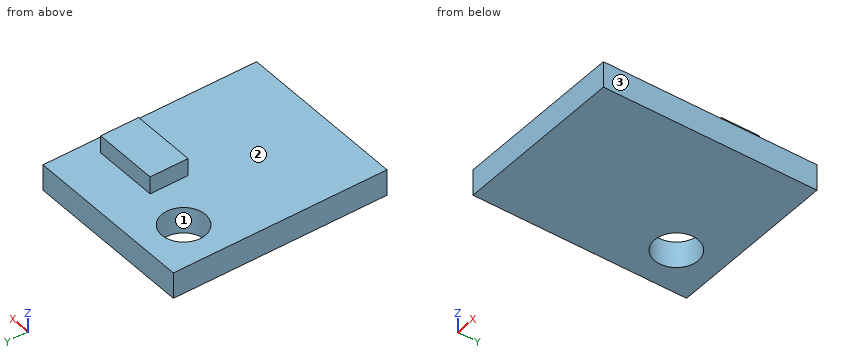
Autodesk Inventor part; units mm, degrees
ref_plane "YZ Plane" through (0, 0, 0) normal (1, 0, 0) x (0, 1, 0)
ref_plane "XZ Plane" through (0, 0, 0) normal (0, 1, 0) x (-1, 0, 0)
ref_plane "XY Plane" through (0, 0, 0) normal (0, 0, 1) x (1, 0, 0)
sketch "Sketch1" plane through (0, 0, 0) normal (0, 0, 1) x (1, 0, 0)
  line L0 (-7.75, 4.08) -> (3.05, 4.08)
  line L1 (3.05, 4.08) -> (3.05, -9.42)
  line L2 (3.05, -9.42) -> (-7.75, -9.42)
  line L3 (-7.75, -9.42) -> (-7.75, 4.08)
  circle A0 centre (-5.025, 1.355) radius 1.375
  line L4 (-2.05, 1.2) -> (2.05, 1.2)
  line L5 (2.05, 1.2) -> (2.05, -1.2)
  line L6 (2.05, -1.2) -> (-2.05, -1.2)
  line L7 (-2.05, -1.2) -> (-2.05, 1.2)
  line L8 (-2.05, 0) -> (2.05, 0)
  line L9 (0, 1.2) -> (0, 0)
  dimension "d0" = 10.8
  dimension "d1" = 13.5
  dimension "d3" = 2.725
  dimension "d4" = 2.75
  dimension "d5" = 4.1
  dimension "d6" = 2.4
  dimension "d8" = 2.88
  dimension "d13" = 1
  dimension "d14" = 2.725
extrude "Extrusion1" add sketch "Sketch1" along normal blind 1.65
extrude "Extrusion2" add sketch "Sketch1" along normal blind 2.75 contours L4 L9 L8 L7 | L4 L5 L8 L9 | L8 L5 L6 L7
properties part number "VL53LDK"
Read the model definition and answer for the solid it produces. Units are mm, in the model's axes. Face numbers are marked on the shaded views. Coordinates: 2 decimals unless noted, no trailing zeros. Loops run counter-clockwise (first coordinate to the right, second up) from the corner with the lowest first, then second, coordinate; pieces in that order, holes last. Notation, with made-up numbers: (4.25, 42.5) - (45.25, 42.5) arc R22 cw to (45.25, 69.5) - close; hole circle Ø6 at (-22.75, 71.5). An arc over 180 degrees is marked (long way). Answer in a Markdown table with one row per item.
1. Find section D-D, the plane y = -1. Write down the section's boundary in (x, z), then the cut area to 3 significant figures.
Conclusion:
| item | result |
|---|---|
| outline | (-7.75, 0) - (3.05, 0) - (3.05, 1.65) - (2.05, 1.65) - (2.05, 2.75) - (-2.05, 2.75) - (-2.05, 1.65) - (-7.75, 1.65) - close |
| area | 22.3 mm² |
2. Find section A-A, the plane x = -1.5. Write down the section's boundary in (y, z), then the cut area to 3 significant figures.
Conclusion:
| item | result |
|---|---|
| outline | (-9.42, 0) - (4.08, 0) - (4.08, 1.65) - (1.2, 1.65) - (1.2, 2.75) - (-1.2, 2.75) - (-1.2, 1.65) - (-9.42, 1.65) - close |
| area | 24.9 mm² |
3. Straight lines are drawn through the part: line 1 (Z direction, x = 0, y = -6); line 2 (Y direction, x = 1.75, z = 1.75); line 3 (X direction, y = -1, z = 2). For each, find the intervals that lie inside material, in ascending order.
Conclusion:
| item | result |
|---|---|
| line 1 | z = 0 to 1.65 |
| line 2 | y = -1.2 to 1.2 |
| line 3 | x = -2.05 to 2.05 |
4. Find section B-B, the plane y = 2. Write down the section's boundary in (x, z), then the cut area to 3 significant figures.
Conclusion:
| item | result |
|---|---|
| outline | (-7.75, 0) - (-6.24, 0) - (-6.24, 1.65) - (-7.75, 1.65) - close; (-3.81, 0) - (3.05, 0) - (3.05, 1.65) - (-3.81, 1.65) - close |
| area | 13.8 mm² |
5. Find section C-C, the plane x = -4. Write down the section's boundary in (y, z), then the cut area to 3 significant figures.
Conclusion:
| item | result |
|---|---|
| outline | (-9.42, 0) - (0.44, 0) - (0.44, 1.65) - (-9.42, 1.65) - close; (2.27, 0) - (4.08, 0) - (4.08, 1.65) - (2.27, 1.65) - close |
| area | 19.3 mm² |
6. Determine the mould class of the marked faces 1, 2 and 3 for opening direction X: +X half, -X half, draft (parallel to the pull), parting line (faces both ways), or undercut.
Conclusion:
| item | result |
|---|---|
| face 1 | undercut |
| face 2 | draft |
| face 3 | +X half |
7. Given pin 1 (4.5 mm diameter, centred on x = -5.025, y = 1.355, fed in from +Z); pin 2 (0.9 mm diameter, centred on y = 0, z = 2.5, fed in from -X); pin 3 (0.6 mm diameter, centred on y = -0.5, z = 2.5, fed in from +X), each flat-ended and moving along its own axis, determine where each tip first touches the part or whether it passes through.
Conclusion:
| item | result |
|---|---|
| pin 1 | stops at z = 1.65 |
| pin 2 | stops at x = -2.05 |
| pin 3 | stops at x = 2.05 |
